from build123d import *

# Parameters (mm, degrees)
REVOLUTION_ANGLE = 180
PAD_DEPTH        = 60
SKETCH002_R      = 3
HOLE_DEPTH       = 131.001
PAD001_DEPTH     = 1.6


with BuildPart() as part:
    # Sketch → Revolution (revolve)
    with BuildSketch(Plane.XZ):
        with BuildLine():
            ThreePointArc((117, 0), (0, 117), (-117, 0))
            Line((-117, 0), (-113, 0))
            ThreePointArc((113, 0), (0, 113), (-113, 0))
            Line((113, 0), (117, 0))
        make_face()
    revolve(axis=Axis((0, 0, 0), (1, 0, 0)), revolution_arc=REVOLUTION_ANGLE)

    # Sketch001 → Pad (new body)
    with BuildSketch(Plane.XZ):
        Polygon((-100, 14), (-100, -14), (-135, -14), (-135, -10), (-122, -10), (-122, 10), (-135, 10), (-135, 14), align=None)
    extrude(amount=PAD_DEPTH)

    # Sketch002 (on Face3 of Pad) → Hole (cut, through all)
    with BuildSketch(Plane(origin=(0, 0, 14), x_dir=(-1, 0, 0), z_dir=(0, 0, 1))):
        with Locations((128.5, 10)):
            Circle(SKETCH002_R)
        with Locations((128.5, 30)):
            Circle(SKETCH002_R)
        with Locations((128.5, 50)):
            Circle(SKETCH002_R)
    extrude(amount=-HOLE_DEPTH, mode=Mode.SUBTRACT)

    # Sketch003 → Pad001 (join)
    with BuildSketch(Plane(origin=(0, 0, 0), x_dir=(1, 0, 0), z_dir=(0, 1, 0))):
        with BuildLine():
            ThreePointArc((-87.124586, -74.345171), (-80.386247, -81.584001), (-73.048555, -88.214548))
            Line((-7.578152, -20.730836), (-73.048555, -88.214548))
            Line((-22.124763, -8.701903), (-7.578152, -20.730836))
            Line((-87.124586, -74.345171), (-22.124763, -8.701903))
        make_face()
        with BuildLine():
            Line((-83.392932, 78.508068), (-21.565299, 11.439582))
            Line((-21.565299, 11.439582), (-9.256599, 22.06979))
            Line((-9.256599, 22.06979), (-71.022068, 89.854125))
            ThreePointArc((-71.022068, 89.854125), (-77.41564, 84.408036), (-83.392932, 78.508068))
        make_face()
        with BuildLine():
            Line((69.065471, 91.366617), (8.92667, 22.06979))
            Line((8.92667, 22.06979), (20.955595, 10.320597))
            Line((20.955595, 10.320597), (81.129513, 80.844913))
            ThreePointArc((81.129513, 80.844913), (75.281537, 86.316789), (69.065471, 91.366617))
        make_face()
        with BuildLine():
            Line((64.925001, -94.353813), (7.527937, -21.849806))
            Line((7.527937, -21.849806), (20.955578, -8.701903))
            Line((20.955578, -8.701903), (80.699204, -81.274451))
            ThreePointArc((64.925001, -94.353813), (73.105196, -88.167614), (80.699204, -81.274451))
        make_face()
    extrude(amount=-PAD001_DEPTH)


solid = part.part
Work out the finished part from the listing and answer in its coordinate system (mm). A direction names the side the tool comes from. Give positions to 0.01 mm unless a question says otherwise; leave off trailing zeros. Loops run counter-clockwise (first coordinate to the right, second up) from the corner with the lowest first, then second, coordinate; pieces in that order, holes last. Notation, with made-up numbers: (41, -13.5) - (46, -13.5) arc R22 cw to (46, 12.5) - close; hole circle Ø8 at (88, 42). An arc over 180 degrees is marked (long way). Answer in a Markdown table with one row per item. Add a question column.
Q1. The part is cut by section D-D (x = -13.5). Determine the outline of the cut face in (y, z).
Q2. Consider line 1 along Y through (x, z) = (-128.5, -12.65); line 2 along X through (y, z) = (-30, -12); line 3 along X through (y, z) = (-50, -11.6). Determine where each line is inside the solid, lowest interval first.
Q3. Each of these flat-tipped pins is pushed along its axis until it touches: P1, Ø10.5, axis at x = -127, y = -16.5, coming from the +Z side; P2, Ø3.5, axis at x = -128.5, y = -10, coming from the -Z side; P3, Ø8, axis at x = -51.5, y = -14.5, coming from the -Z side; P4, Ø8, axis at y = -67, z = 85.5, coming from the +X side. Where does it stop, or does it pass through?
Q4. A tool of negligible diameter and unlimited length cuts with its end or side. For faces 1 (the flat face through (-122, -36, 14)), 2 (the flat face through (-133, -30, -10)), 3 (the flat face through (-100, -26, 0)), from which of +Z, -Z, +X, -X, +Y, -Y can it reach the whole face along a straight path? Write none if from no direction.
Q5. The part is cut by section B-B (y = -30). Determine the outline of the cut face in (x, z), and give its area (3 significant figures).
Q6. Determine the mould class of faces 4 (the flat face through (-39.33, -0.79, 53.46)), 5 (the flat face through (-18, 0, 27)), 6 (the flat face through (-122, -30, 0)), 7 (the flat face through (-49, -1.6, -50)) for opening direction X: released by +X, released by -X, zero draft, split by the parting line, or undercut.
Q7. The part is cut by section C-C (z = 54.5). Determine the outline of the cut face in (x, y), and give its area (3 significant figures).
Q8. The part is cut by section A-A (x = -128.5). State how many separate pieces and enclosed holes the cut face has, and give its area (3 significant figures).
Solution:
| question | item | result |
|---|---|---|
| 1 | outline | (-1.6, -26.73) - (0, -26.73) - (0, -18.41) - (-1.6, -18.41) - close; (-1.6, 15.83) - (0, 15.83) - (0, 26.83) - (-1.6, 26.83) - close; (0, -116.22) - (0, -112.19) arc R112.19 cw to (0, 112.19) - (0, 116.22) arc R116.22 ccw to start |
| 2 | line 1 | y = -60 to -53, -47 to -33, -27 to -13, -7 to 0 |
| 2 | line 2 | x = -135 to -131.5, -125.5 to -100, 108.28 to 112.45 |
| 2 | line 3 | x = -135 to -131.5, -125.5 to -100, 100.67 to 105.14 |
| 3 | P1 | stops at z = 14 |
| 3 | P2 | passes through |
| 3 | P3 | stops at z = -106.01 |
| 3 | P4 | stops at x = 52.37 |
| 4 | face 1 | +Z, -X, -Y |
| 4 | face 2 | -X, +Y, -Y |
| 4 | face 3 | +Y |
| 5 | outline | (-135, -14) - (-131.5, -14) - (-131.5, -10) - (-135, -10) - close; (-135, 10) - (-131.5, 10) - (-131.5, 14) - (-135, 14) - close; (-125.5, -14) - (-112.22, -14) arc R113.09 ccw (long way) to (-112.22, 14) - (-125.5, 14) - (-125.5, 10) - (-122, 10) - (-122, -10) - (-125.5, -10) - close; hole (-108.04, -14) arc R108.94 ccw (long way) to (-108.04, 14) - (-100, 14) - (-100, -14) - close |
| 5 | area | 3,450 mm² |
| 6 | face 4 | undercut |
| 6 | face 5 | zero draft |
| 6 | face 6 | released by -X |
| 6 | face 7 | undercut |
| 7 | outline | (-103.53, 0) arc R103.53 ccw to (103.53, 0) - (98.99, 0) arc R98.99 cw to (-98.99, 0) - close; (-67.47, -1.6) - (-40.34, -1.6) - (-40.34, 0) - (-67.47, 0) - close; (33.38, -1.6) - (58.66, -1.6) - (58.66, 0) - (33.38, 0) - close |
| 7 | area | 1,530 mm² |
| 8 | separate pieces | 8 |
| 8 | enclosed holes | 0 |
| 8 | area | 336 mm² |
